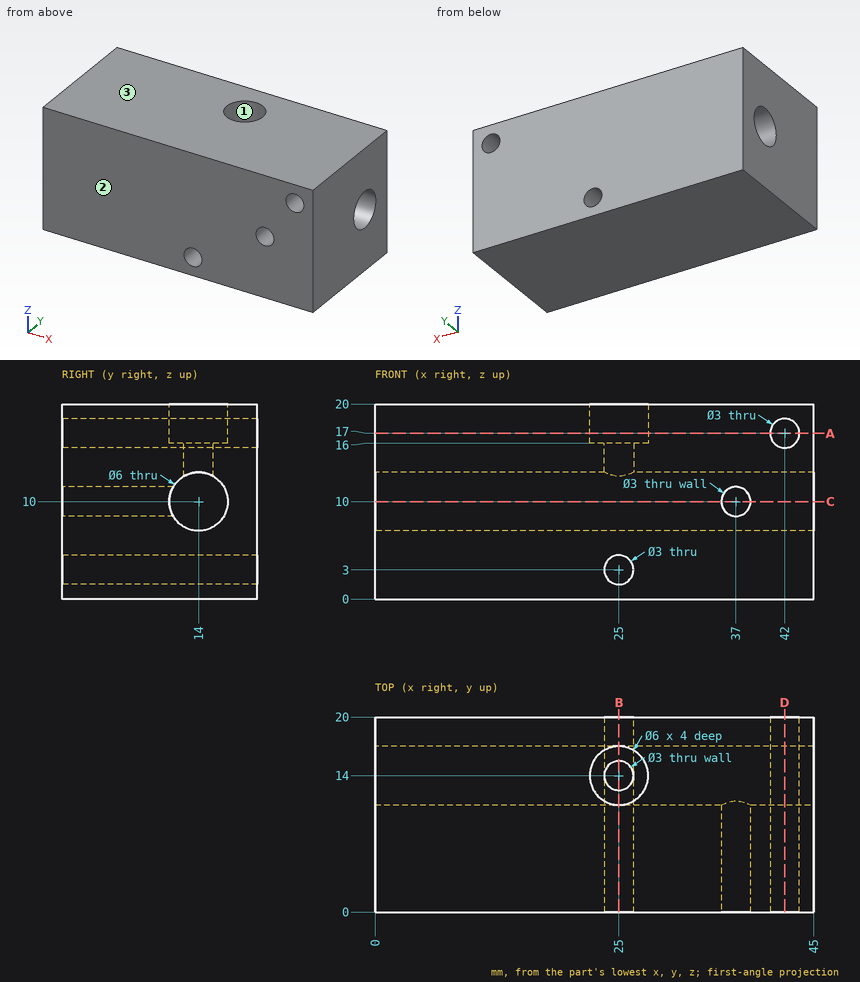
Answer from the drawing. Dimensions are ordinates in mm from the lowest x, y and z of the part. Coordinates: 2 decimals unless noted, no trailing zeros. Loops run counter-clockwise (first coordinate to the right, second up) from the corner with the lowest first, then second, coordinate; pieces in that order, holes last. Notation, with made-up numbers: (4.25, -20) - (25.25, -20) arc R10 ccw to (25.25, -12) - close; hole circle Ø9 at (-35.5, 26.5). An arc over 180 degrees is marked (long way). Answer in a Markdown table with one row per item.
1. Find section B-B, the plane x = 25. Write down the section's boundary in (y, z), then the cut area to 3 significant figures.
Conclusion:
| item | result |
|---|---|
| outline | (0, 0) - (20, 0) - (20, 1.5) - (0, 1.5) - close; (0, 4.5) - (20, 4.5) - (20, 20) - (17, 20) - (17, 16) - (15.5, 16) - (15.5, 12.6) arc R3 cw (long way) to (12.5, 12.6) - (12.5, 16) - (11, 16) - (11, 20) - (0, 20) - close |
| area | 278 mm² |
2. Determine the mould class of the marked faces 1, 2 and 3 for opening direction Y: +Y half, -Y half, draft (parallel to the pull), parting line (faces both ways), or undercut.
Conclusion:
| item | result |
|---|---|
| face 1 | undercut |
| face 2 | -Y half |
| face 3 | draft |
3. Find section D-D, the plane x = 42. Write down the section's boundary in (y, z), then the cut area to 3 significant figures.
Conclusion:
| item | result |
|---|---|
| outline | (0, 0) - (20, 0) - (20, 15.5) - (0, 15.5) - close; (0, 18.5) - (20, 18.5) - (20, 20) - (0, 20) - close; hole circle Ø6 at (14, 10) |
| area | 312 mm² |
4. Find section A-A, the plane z = 17. Write down the section's boundary in (x, y), then the cut area to 3 significant figures.
Conclusion:
| item | result |
|---|---|
| outline | (0, 0) - (40.5, 0) - (40.5, 20) - (0, 20) - close; (43.5, 0) - (45, 0) - (45, 20) - (43.5, 20) - close; hole circle Ø6 at (25, 14) |
| area | 812 mm² |
5. Given pin 1 (9.5 mm diameter, centred on y = 14, z = 10, fed in from +X); pin 2 (1.8 mm diameter, centred on x = 26, y = 13, fed in from +Z); pin 3 (2.5 mm diameter, centred on x = 42, z = 17, fed in from +Y), each flat-ended and moving along its own axis, determine where each tip first touches the part or whether it passes through.
Conclusion:
| item | result |
|---|---|
| pin 1 | stops at x = 45 |
| pin 2 | stops at z = 16 |
| pin 3 | passes through |
6. Straight lines are drawn through the part: line 1 (Z direction, x = 42, y = 9); line 2 (Y direction, x = 32.5, z = 9.75); line 3 (Z direction, x = 11.5, y = 13.75). For each, find the intervals that lie inside material, in ascending order.
Conclusion:
| item | result |
|---|---|
| line 1 | z = 0 to 15.5, 18.5 to 20 |
| line 2 | y = 0 to 11.01, 16.99 to 20 |
| line 3 | z = 0 to 7.01, 12.99 to 20 |
7. Find section C-C, the plane z = 10. Write down the section's boundary in (x, y), then the cut area to 3 significant figures.
Conclusion:
| item | result |
|---|---|
| outline | (0, 0) - (35.5, 0) - (35.5, 11) - (0, 11) - close; (0, 17) - (45, 17) - (45, 20) - (0, 20) - close; (38.5, 0) - (45, 0) - (45, 11) - (38.5, 11) - close |
| area | 597 mm² |
